from build123d import *

# Parameters (mm, degrees)
F0_W      = 200
F0_H      = 50
F1_DEPTH  = 10
F2_W      = 42
F2_H      = 22
F3_DEPTH  = 10.001
F5_DEPTH  = 10.001
F7_DEPTH  = 10.001
F8_R      = 5
F11_W     = 80
F11_H     = 20
F9_W      = 12.4
F9_H      = 11.4
F12_DEPTH = 10.001
F13_R     = 5


with BuildPart() as f1:
    # F0 (on Top) → F1 (new body)
    with BuildSketch(Plane.XY):
        Rectangle(F0_W, F0_H)
    extrude(amount=F1_DEPTH)

    # F2 (on face) → F3 (cut, through all)
    with BuildSketch(Plane.XY.offset(10)):
        with Locations((-57.7500068545, -5)):
            Rectangle(F2_W, F2_H)
    extrude(amount=-F3_DEPTH, mode=Mode.SUBTRACT)

    # F4 (on face) → F5 (cut, through all)
    with BuildSketch(Plane.XY.offset(10)):
        with BuildLine():
            Line((-81.6500068545, -2.15), (-81.6500068545, 0.1))
            Line((-81.6500068545, 0.1), (-79.4000068545, 0.1))
            ThreePointArc((-79.4000068545, 0.1), (-83.2409971122, 1.6909902577), (-81.6500068545, -2.15))
        make_face()
        with BuildLine():
            Line((-79.4000068545, 0.1), (-81.6500068545, 0.1))
            Line((-81.6500068545, 0.1), (-81.6500068545, -2.15))
            ThreePointArc((-81.6500068545, -2.15), (-80.0590165969, -1.4909902577), (-79.4000068545, 0.1))
        make_face()
        with BuildLine():
            Line((-81.6500068545, -10.1), (-81.6500068545, -7.85))
            ThreePointArc((-81.6500068545, -7.85), (-83.2409971122, -11.6909902577), (-79.4000068545, -10.1))
            Line((-79.4000068545, -10.1), (-81.6500068545, -10.1))
        make_face()
        with BuildLine():
            ThreePointArc((-79.4000068545, -10.1), (-80.0590165969, -8.5090097423), (-81.6500068545, -7.85))
            Line((-81.6500068545, -7.85), (-81.6500068545, -10.1))
            Line((-81.6500068545, -10.1), (-79.4000068545, -10.1))
        make_face()
        with BuildLine():
            Line((-33.8500068545, 0.1), (-36.1000068545, 0.1))
            ThreePointArc((-36.1000068545, 0.1), (-35.4409971122, -1.4909902577), (-33.8500068545, -2.15))
            Line((-33.8500068545, -2.15), (-33.8500068545, 0.1))
        make_face()
        with BuildLine():
            ThreePointArc((-31.6000068545, 0.1), (-33.8500068545, 2.35), (-36.1000068545, 0.1))
            Line((-36.1000068545, 0.1), (-33.8500068545, 0.1))
            Line((-33.8500068545, 0.1), (-33.8500068545, -2.15))
            ThreePointArc((-33.8500068545, -2.15), (-32.2590165969, -1.4909902577), (-31.6000068545, 0.1))
        make_face()
        with BuildLine():
            ThreePointArc((-33.8500068545, -7.85), (-35.4409971122, -8.5090097423), (-36.1000068545, -10.1))
            Line((-36.1000068545, -10.1), (-33.8500068545, -10.1))
            Line((-33.8500068545, -10.1), (-33.8500068545, -7.85))
        make_face()
        with BuildLine():
            Line((-33.8500068545, -10.1), (-36.1000068545, -10.1))
            ThreePointArc((-36.1000068545, -10.1), (-33.8500068545, -12.35), (-31.6000068545, -10.1))
            ThreePointArc((-31.6000068545, -10.1), (-32.2590165969, -8.5090097423), (-33.8500068545, -7.85))
            Line((-33.8500068545, -7.85), (-33.8500068545, -10.1))
        make_face()
    extrude(amount=-F5_DEPTH, mode=Mode.SUBTRACT)

    # F6 (on face) → F7 (cut, through all)
    with BuildSketch(Plane.XY.offset(10)):
        with BuildLine():
            Line((-87.8187507391, 11.5), (-87.8187507391, 15))
            Line((-87.8187507391, 15), (-84.3187507391, 15))
            ThreePointArc((-84.3187507391, 15), (-90.2936244733, 17.4748737342), (-87.8187507391, 11.5))
        make_face()
        with BuildLine():
            Line((-84.3187507391, 15), (-87.8187507391, 15))
            Line((-87.8187507391, 15), (-87.8187507391, 11.5))
            ThreePointArc((-87.8187507391, 11.5), (-85.3438770049, 12.5251262658), (-84.3187507391, 15))
        make_face()
        with BuildLine():
            Line((-7.8187507391, 15), (-11.3187507391, 15))
            ThreePointArc((-11.3187507391, 15), (-10.2936244733, 12.5251262658), (-7.8187507391, 11.5))
            Line((-7.8187507391, 11.5), (-7.8187507391, 15))
        make_face()
        with BuildLine():
            ThreePointArc((-4.3187507391, 15), (-7.8187507391, 18.5), (-11.3187507391, 15))
            Line((-11.3187507391, 15), (-7.8187507391, 15))
            Line((-7.8187507391, 15), (-7.8187507391, 11.5))
            ThreePointArc((-7.8187507391, 11.5), (-5.3438770049, 12.5251262658), (-4.3187507391, 15))
        make_face()
    extrude(amount=-F7_DEPTH, mode=Mode.SUBTRACT)

    # F8
    f8_edges = [f1.edges().sort_by_distance(p)[0] for p in [
        (-100, 25, 5),
        (-100, -25, 5),
        (100, 25, 5),
        (100, -25, 5),
    ]]
    fillet(f8_edges, radius=F8_R)

    # F11 (on face) + F10 (on face) + F9 (on face) → F12 (cut, through all)
    with BuildSketch(Plane.XY.offset(10)):
        with Locations((60, 15)):
            Rectangle(F11_W, F11_H)
    with BuildSketch(Plane.XY.offset(10)):
        with BuildLine():
            ThreePointArc((93.6749931455, -5), (91.2499931455, -2.575), (88.8249931455, -5))
            Line((88.8249931455, -5), (91.2499931455, -5))
            Line((91.2499931455, -5), (91.2499931455, -7.425))
            ThreePointArc((91.2499931455, -7.425), (92.9647270898, -6.7147339444), (93.6749931455, -5))
        make_face()
        with BuildLine():
            Line((91.2499931455, -5), (88.8249931455, -5))
            ThreePointArc((88.8249931455, -5), (89.5352592011, -6.7147339444), (91.2499931455, -7.425))
            Line((91.2499931455, -7.425), (91.2499931455, -5))
        make_face()
    with BuildSketch(Plane.XY.offset(10)):
        with Locations((6.2, -12.7)):
            Rectangle(F9_W, F9_H)
    extrude(amount=-F12_DEPTH, mode=Mode.SUBTRACT)

    # F13
    f13_edges = [f1.edges().sort_by_distance(p)[0] for p in [
        (20, 25, 5),
        (20, 5, 5),
        (100, 5, 5),
    ]]
    fillet(f13_edges, radius=F13_R)


solid = f1.part
Work out the finished part from the listing and answer in its coordinate system (mm). A direction names the side the tool comes from. Round coordinates to 2 decimals unless told otherwise and drop trailing zeros. Loops run counter-clockwise (first coordinate to the right, second up) from the corner with the lowest first, then second, coordinate; pieces in that order, holes last. Notation, with made-up numbers: M 61.25,-24 L 90.25,-24 A25 ccw 90.25,-2 Z; hole C 4,56.25 d2. An arc over 180 degrees is marked long. One line per question, with ' | ' between items. Start each with the question number.
(1) A cutting plane is placed at A-A on x = -58. Write down the section's boundary in (y, z), plus the area to 3 significant figures.
(2) A tool of negligible diameter and unlimited length cuts with its end or side. For faces 1 (the face through (20, 15, 5)), 2 (the face through (12.4, -13, 5)), 3 (the face through (98, -24, 5)), from which of +Z, -Z, +X, -X, +Y, -Y can it reach the whole face along a straight path? Write none if from no direction.
(3) Flat-ended cylindrical pins translate along their axes: pin 1 Ø4 at (x, y) = (-81.65, 0.1) entering from +Z; pin 2 Ø6 at (x, z) = (26, 8.5) entering from +Y; pin 3 Ø5 at (y, z) = (14, 4) entering from +X. Find the tip coordinate at first contact, or state that the pin passes through.
(4) A cutting plane is placed at C-C on x = 70.5. Write down the section's boundary in (y, z).
(5) For a pull along Y with two mould halves and no side action, classify faces 4 (the face through (6, -7, 5)), 5 (the face through (-41, 25, 5)), 6 (the face through (-1, -25, 5)), 7 (the face through (100, -10, 5)) as released by +Y, released by -Y, zero draft, split by the parting line, or undercut.
(6) Find the intervals of material crossed by line 1 (X direction, y = -14, z = 9.25); line 2 (X direction, y = -5, z = 9) (3 decimals); line 3 (X direction, y = -10.1, z = 6.5), in increasing order.
(7) A cutting plane is placed at B-B on z = 2.75. Give the number of separate pieces and of enclosed holes in the cut face, plus the area to 3 significant figures.
Geometry check:
1) outline: M -25,0 L -16,0 L -16,10 L -25,10 Z; M 6,0 L 25,0 L 25,10 L 6,10 Z | area: 280 mm²
2) face 1: +Z, -Z, +X, +Y | face 2: +Z, -Z | face 3: +Z, -Z, +X, -Y
3) pin 1: passes through | pin 2: stops at y = 5.42 | pin 3: stops at x = 20
4) outline: M -25,0 L 5,0 L 5,10 L -25,10 Z
5) face 4: undercut | face 5: released by +Y | face 6: released by -Y | face 7: zero draft
6) line 1: x = -100 to -78.75, -36.75 to 0, 12.4 to 100 | line 2: x = -100 to -78.75, -36.75 to 88.825, 93.675 to 100 | line 3: x = -100 to -83.9, -79.4 to -78.75, -36.75 to -36.1, -31.6 to 0, 12.4 to 100
7) separate pieces: 1 | enclosed holes: 9 | area: 7,150 mm²
